Input: dimensioned drawing with shaded views. Units: mm. Origin: part minimum x, y, z. Give positions to 0.01 mm unless a question says otherwise; leave off trailing zeros. Loops run counter-clockwise (first coordinate to the right, second up) from the corner with the lowest first, then second, coordinate; pieces in that order, holes last.
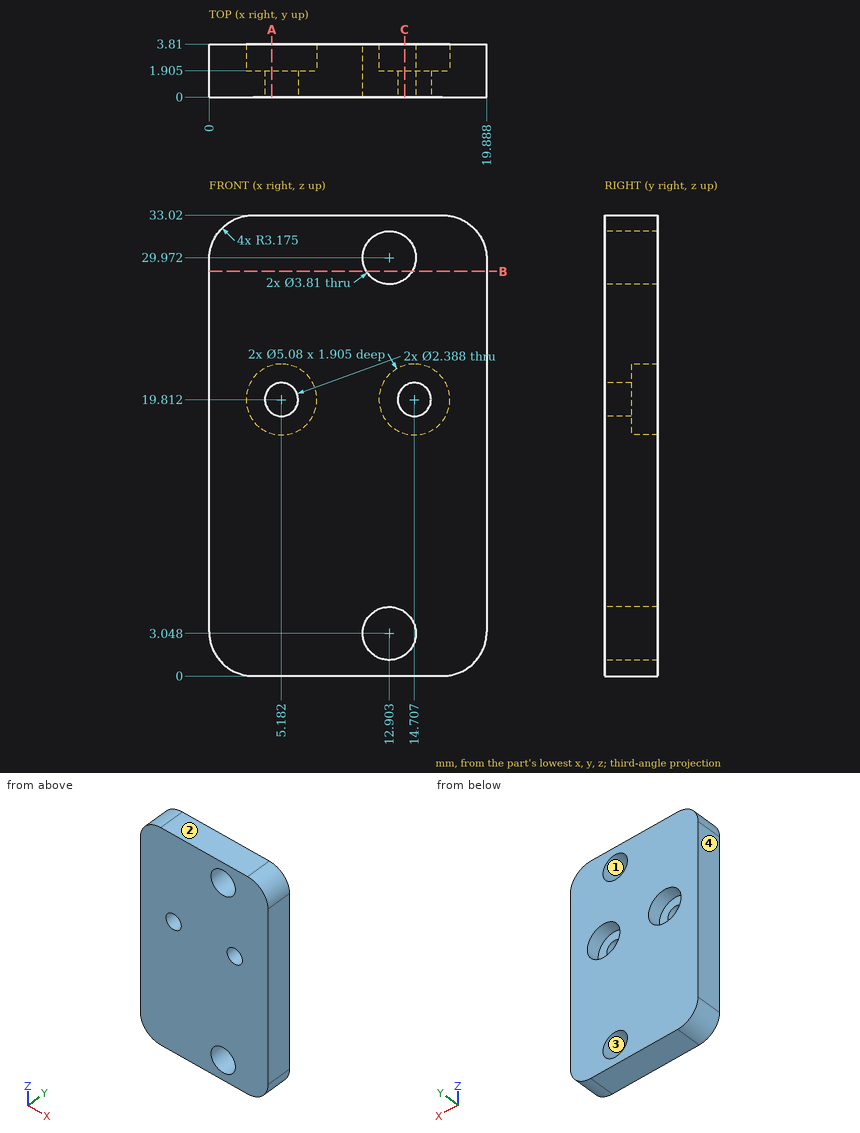
(1) Section B-B, the plane z = 29. Return the cut outline in (x, y) (1 decimal), then the cut area to 3 significant figures.
A:
outline: (0, 0) - (11.3, 0) - (11.3, 3.8) - (0, 3.8) - close; (14.5, 0) - (19.9, 0) - (19.9, 3.8) - (14.5, 3.8) - close
area: 63.3 mm2
(2) Mould query, pull axis Z, two halves, no side actions, for the marked faces 1, 2, 3 and 4. Classes: pulls with the +Z half, pulls with the -Z half, needs draft (parallel to the pull), parting line crosses it, or undercut.
A:
face 1: undercut
face 2: pulls with the +Z half
face 3: undercut
face 4: needs draft
(3) First-contact query: pin 1 (1.5 mm diameter, centred on x = 13.5, z = 19, fed in from +Y) (3 decimals). Flat tip, straight axial feed; report the tip coordinate or a pass-through.
A:
pin 1: stops at y = 1.905
(4) Section C-C, the plane x = 14. Count the separate pieces of the cut face and the enclosed holes in it.
A:
separate pieces: 4
enclosed holes: 0
(5) Ray query, line 1 along X through (y, z) = (2.85, 20) (1 decimal); line 2 along Z through (x, y) = (11.75, 1.9) (1 decimal); line 3 along Z through (x, y) = (14.5, 0.9) (1 decimal). Return the intervals inside material, ascending.
A:
line 1: x = 0 to 2.6, 7.7 to 12.2, 17.2 to 19.9
line 2: z = 0 to 1.5, 4.6 to 28.5, 31.5 to 33
line 3: z = 0 to 2, 4.1 to 18.6, 21 to 28.9, 31 to 33
(6) Section A-A, the plane x = 4.5. Return the cut outline in (y, z) (1 decimal), then the cut area to 3 significant figures.
A:
outline: (0, 0) - (3.8, 0) - (3.8, 17.4) - (1.9, 17.4) - (1.9, 18.8) - (0, 18.8) - close; (0, 20.8) - (1.9, 20.8) - (1.9, 22.3) - (3.8, 22.3) - (3.8, 33) - (0, 33) - close
area: 113 mm2
